Input: part model. Units: mm. Frame: model coordinates. Give positions to 0.01 mm unless a question says otherwise; leave off trailing zeros. Order: outer loops, then holes, each group sorted by start corner. A loop starts at its lowest first (then second) coordinate and runs counter-clockwise, first axis right, second up. Notation, with made-up numbers: (45, -9) - (73, -9) arc R24 cw to (73, 15) - close; hole circle Ø4 at (36, 48). An arc over 180 degrees is marked (long way). Answer in a Markdown table with one row per item. Add a question column.
from build123d import *

# Parameters (mm, degrees)
F0_R     = 1.75
F0_W     = 12.5
F0_H     = 11.2
F0_R_2   = 1.6
F0_R_3   = 11
F0_W_2   = 9.4
F1_DEPTH = 2


with BuildPart() as f1:
    # F0 (on Top) → F1 (new body)
    with BuildSketch(Plane.XY):
        Polygon((124.39022, 20.678444), (-108.10978, 20.678444), (-114.60978, 14.178444), (-114.60978, -18.321556), (-108.10978, -24.821556), (124.39022, -24.821556), (130.89022, -18.321556), (130.89022, 14.178444), align=None)
        with Locations((-107.35978, -17.571556)):
            Circle(F0_R, mode=Mode.SUBTRACT)
        with Locations((-107.35978, 13.428444)):
            Circle(F0_R, mode=Mode.SUBTRACT)
        with Locations((34.64022, -8.971556)):
            Rectangle(F0_W, F0_H, mode=Mode.SUBTRACT)
        with Locations((65.29022, -11.971556)):
            Circle(F0_R_2, mode=Mode.SUBTRACT)
        with Locations((45.49022, 7.828444)):
            Circle(F0_R_2, mode=Mode.SUBTRACT)
        with Locations((55.39022, -2.071556)):
            Circle(F0_R_3, mode=Mode.SUBTRACT)
        with Locations((84.39022, -8.971556)):
            Rectangle(F0_W_2, F0_H, mode=Mode.SUBTRACT)
        with Locations((123.64022, -17.571556)):
            Circle(F0_R, mode=Mode.SUBTRACT)
        with Locations((123.64022, 13.428444)):
            Circle(F0_R, mode=Mode.SUBTRACT)
    extrude(amount=F1_DEPTH)


solid = f1.part
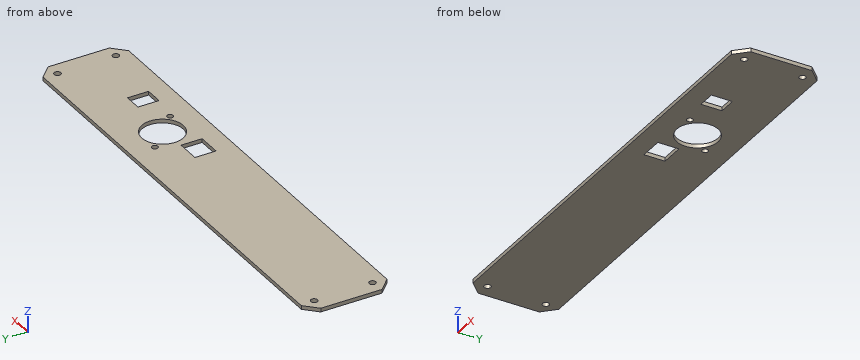
Q1. Line query: probe 1 along X at (y, z) = (13.5, 0.2); probe 2 along Y at (x, z) = (81, 1.95); probe 3 along X at (y, z) = (12, 0.3). Output: solid intervals per line, ascending.
Q2. Section C-C, the plane z = 0.3. State how many separate pieces and enclosed holes the cut face has, then the cut area to 3 significant figures.
Q3. Section A-A, the plane x = 82. Return loops of the section in (y, z).
Q4. Section B-B, the plane y = 1. Return loops of the section in (x, z).
Computed:
| question | item | result |
|---|---|---|
| 1 | probe 1 | x = -114.61 to -109.11, -105.61 to 121.89, 125.39 to 130.89 |
| 1 | probe 2 | y = -24.82 to -14.57, -3.37 to 20.68 |
| 1 | probe 3 | x = -114.61 to -108.37, -106.35 to 122.63, 124.65 to 130.89 |
| 2 | separate pieces | 1 |
| 2 | enclosed holes | 9 |
| 2 | area | 10,400 mm^2 |
| 3 | outline | (-24.82, 0) - (-14.57, 0) - (-14.57, 2) - (-24.82, 2) - close; (-3.37, 0) - (20.68, 0) - (20.68, 2) - (-3.37, 2) - close |
| 4 | outline | (-114.61, 0) - (44.83, 0) - (44.83, 2) - (-114.61, 2) - close; (65.95, 0) - (130.89, 0) - (130.89, 2) - (65.95, 2) - close |
